from build123d import *

# Parameters (mm, degrees)
BASETOP_FACE_RADIUS = 2.6
BASETOP_HEIGHT      = 0.7
CROSSRECESS_DEPTH   = 0.825
DRAFT9_ANGLE        = -30
FILLET5_R           = 0.3


with BuildPart() as part:
    # Sketch1 → Base (revolve)
    with BuildSketch(Plane.XY):
        Polygon((16, 1.5), (2.737867966, 1.5), (1.467367966, 1.5), (0.367367966, 2.6), (0, 2.6), (0, 0), (16, 0), align=None)
    revolve(axis=Axis((4.515812911, 0, 0), (-1, 0, 0)))

    # BaseTop: a dome of height H over a round flat face of radius A is a cap of a sphere of radius (A * A + H * H) / (2 * H)
    basetop_r = (BASETOP_FACE_RADIUS * BASETOP_FACE_RADIUS + BASETOP_HEIGHT * BASETOP_HEIGHT) / (2 * BASETOP_HEIGHT)
    basetop_base = Plane((0, 0, 0), z_dir=(-1, 0, 0))
    with Locations(basetop_base.offset(BASETOP_HEIGHT - basetop_r)):
        basetop_ball = Sphere(basetop_r, mode=Mode.PRIVATE)
    add(split(basetop_ball, bisect_by=basetop_base, keep=Keep.TOP, mode=Mode.PRIVATE))

    # Sketch6 → CrossRecess (cut)
    with BuildSketch(Plane.ZY.offset(0.7)):
        Polygon((0.34, 0.34), (0.34, 1.7), (-0.34, 1.7), (-0.34, 0.34), (-1.7, 0.34), (-1.7, -0.34), (-0.34, -0.34), (-0.34, -1.7), (0.34, -1.7), (0.34, -0.34), (1.7, -0.34), (1.7, 0.34), align=None)
    extrude(amount=-CROSSRECESS_DEPTH, mode=Mode.SUBTRACT)

    # Draft9
    draft9_faces = [part.faces().sort_by_distance(p)[0] for p in [
        (-0.14204754, 0, -1.7),
        (-0.14204754, -1.7, 0),
        (-0.14204754, 0, 1.7),
        (-0.14204754, 1.7, 0),
    ]]
    draft(draft9_faces, Plane(origin=(-0.7, 0, 0), x_dir=(0, 0, 1), z_dir=(1, 0, 0)), DRAFT9_ANGLE)

    # Fillet5
    fillet5_edges = [part.edges().sort_by_distance(p)[0] for p in [
        (-0.27631446, 0.34, -0.34),
        (-0.27631446, 0.34, 0.34),
        (-0.27631446, -0.34, 0.34),
        (-0.27631446, -0.34, -0.34),
    ]]
    fillet(fillet5_edges, radius=FILLET5_R)


solid = part.part
Source: CAD feature listing. Evaluate the final solid. Frame: model axes, mm. Coordinates: 2 decimals unless noted, no trailing zeros. Loops run counter-clockwise (first coordinate to the right, second up) from the corner with the lowest first, then second, coordinate; pieces in that order, holes last. Notation, with made-up numbers: M 35.5,65.5 L 53.5,65.5 A17 cw 53.5,87.5 Z; hole C 70.25,56 d10. An arc over 180 degrees is marked long. Answer in a Markdown table with one row per item.
Q1. Draft query along Z for faces 1 (the flat face through (0.125, 0, 0)), 2 (the cylindrical face through (8.63, -1.5, -0.07)), 3 (the flat face through (16, 0, 0)). Return one class per face: pulls with the +Z half, pulls with the -Z half, needs draft (parallel to the pull), parting line crosses it, or undercut.
Answers below:
| item | result |
|---|---|
| face 1 | undercut |
| face 2 | parting line crosses it |
| face 3 | needs draft |
Q2. First-contact query: pin 1 (2 mm diameter, centred on y = 0, z = -1, fed in from -X); pin 2 (3 mm diameter, centred on x = 3, z = 0, fed in from -Y); pin 3 (0.9 mm diameter, centred on x = 0, z = 1, fed in from -Y); pin 4 (3 mm diameter, centred on x = 7, y = -1, fed in from -Z). Flat tips, straight axial feed; report the tip coordinate or a pass-through.
Answers below:
| item | result |
|---|---|
| pin 1 | stops at x = -0.66 |
| pin 2 | stops at y = -1.5 |
| pin 3 | stops at y = -2.54 |
| pin 4 | stops at z = -1.5 |
Q3. Section A-A on y = 0. Return the cut outline in (x, z) (3 decimals).
Answers below:
| item | result |
|---|---|
| outline | M -0.459,-1.561 A5.179 ccw 0,-2.6 L 0.367,-2.6 L 1.467,-1.5 L 16,-1.5 L 16,1.5 L 1.467,1.5 L 0.367,2.6 L 0,2.6 A5.179 ccw -0.459,1.561 L 0.125,1.224 L 0.125,-1.224 Z |
Q4. Section C-C on x = 9.5. Return the cut outline in (y, z), plus the area to 3 significant figures.
Answers below:
| item | result |
|---|---|
| outline | C 0,0 d3 |
| area | 7.07 mm^2 |
Q5. Ray query, probe 1 along Y at (x, z) = (14, -0.1); probe 2 along X at (y, z) = (0.65, 0.6); probe 3 along X at (y, z) = (-0.9, 1.6). Return the intervals inside material, ascending. Write a range as from..to.
Answers below:
| item | result |
|---|---|
| probe 1 | y = -1.5..1.5 |
| probe 2 | x = -0.62..16 |
| probe 3 | x = -0.36..1.13 |
Q6. Section D-D on x = 0.75. Return the cut outline in (y, z).
Answers below:
| item | result |
|---|---|
| outline | C 0,0 d4.43 |
